Autodesk Inventor part; units mm, degrees
ref_plane "Work Plane1" through (0, 20, 0) normal (0, 1, 0) x (-1, 0, 0)
ref_plane "Work Plane3" through (0, 0, 0) normal (-1, 0, 0) x (0, 0, 1)
ref_plane "YZ Plane" through (0, 0, 0) normal (1, 0, 0) x (0, 1, 0)
sketch "Sketch1" plane through (0, 0, 0) normal (0, 0, 1) x (1, 0, 0)
  line L0 (0, 0) -> (0, 6.5)
  line L1 (0, 6.5) -> (55, 6.5)
  line L2 (68, 1.75) -> (55, 6.5)
  line L3 (72, 0) -> (72, 2.5)
  line L4 (72, 2.5) -> (68, 1.75)
  line L5 (0, 6.5) -> (0, 9.5)
  line L6 (0, 9.5) -> (60.7761, 9.5)
  line L7 (72, 0) -> (0, 0)
  line L8 (72, 2.5) -> (72, 4.5)
  line L9 (72, 4.5) -> (66.9088, 4.5)
  line L10 (66.9088, 4.5) -> (66.9088, 9.5)
  line L11 (66.9088, 9.5) -> (60.7761, 9.5)
  line L12 (66.9088, 9.5) -> (66.9088, 9.5)
  line L13 (66.9088, 9.5) -> (16.9088, 9.5)
  line L14 (16.9088, 9.5) -> (16.9088, 9.5)
  point P0 (72, 1.25)
  dimension "d0" = 6.5
  dimension "d1" = 55
  dimension "d5" = 2.5
  dimension "d6" = 3
  dimension "d7" = 0
  dimension "d8" = 50
  dimension "d44" = 1.75
  dimension "d45" = 4
  dimension "d46" = 13
revolve "Revolution1" add sketch "Sketch1" angle 360 about axis through (72, 0, 0) along (-1, 0, 0) contours L5 L6 L11 L10 L9 L8 L4 L2 L1
sketch "Sketch2" plane through (0, 0, 0) normal (-1, 0, 0) x (0, 0, 1)
  circle A0 centre (0, 0) radius 2.5
  circle A1 centre (0, 0) radius 20
  circle A2 centre (0, 0) radius 6.5
  dimension "d10" = 40
  dimension "d11" = 13
extrude "Extrusion1" add sketch "Sketch2" along normal blind 19 contours A1
sketch "Sketch3" plane through (0, 0, 0) normal (1, 0, 0) x (0, 0, -1)
  circle A0 centre (0, 0) radius 1.75
  circle A1 centre (0, 0) radius 20
  circle A2 centre (0, 0) radius 4.5
  circle A3 centre (0, 0) radius 9.5
  dimension "d18" = 40
  dimension "d37" = 19
extrude "Extrusion2" add sketch "Sketch3" along normal blind 15 contours A1
sketch "Sketch4" plane through (0, 0, 0) normal (0, 1, 0) x (-1, 0, 0)
  line L0 (19, -20) -> (19, 20)
  line L1 (19, 0) -> (-5, 0)
  circle A0 centre (-5, 0) radius 1.75
  point P0 (0, 0)
  dimension "d21" = 24
  dimension "d22" = 3.5
extrude "Extrusion3" cut sketch "Sketch4" along normal through all both and the other way through all
ref_plane "Work Plane1" through (0, 20, 0) normal (0, 1, 0) x (-1, 0, 0)
sketch "Sketch5" plane through (0, 20, 0) normal (0, 1, 0) x (-1, 0, 0)
  line L0 (19, -20) -> (19, 20)
  line L1 (19, 0) -> (-5, 0)
  circle A0 centre (-5, 0) radius 3.175
  point P0 (0, 0)
  dimension "d26" = 24
  dimension "d27" = 6.35
hole "Hole1" at (5, 20, 0) direction (0, -1, 0) diameter 2 end through all counterbore diameter 11 counterbore depth 6
thread "Thread3"
mirror "Mirror1" about plane through (0, 0, 0) normal (0, 1, 0) of "Hole1"
thread "Thread4"
ref_plane "Work Plane3" through (0, 0, 0) normal (-1, 0, 0) x (0, 0, 1)
ref_plane "Work Plane2" through (0, 0, 0) normal (0, 1, 0) x (-1, 0, 0)
properties part number "ASI Propane" material "Stainless Steel"
Read the model definition and answer for the solid it produces. Units are mm, in the model's axes. A direction names the side the tool comes from. Coordinates: 2 decimals unless noted, no trailing zeros. Loops run counter-clockwise (first coordinate to the right, second up) from the corner with the lowest first, then second, coordinate; pieces in that order, holes last.
(1) The part is cut by section A-A (x = 5). Determine the outline of the cut face in (y, z).
Solution:
outline: (-19.23, -5.5) arc R20 ccw to (19.23, -5.5) - (14, -5.5) - (14, -1.75) - (6.26, -1.75) arc R6.5 cw to (-6.26, -1.75) - (-14, -1.75) - (-14, -5.5) - close; (-19.23, 5.5) - (-14, 5.5) - (-14, 1.75) - (-6.26, 1.75) arc R6.5 cw to (6.26, 1.75) - (14, 1.75) - (14, 5.5) - (19.23, 5.5) arc R20 ccw to start
(2) The mould has two halves that part along Y. Classify faces 1 (the face through (-2.238, 19.956, 1.319)), 2 (the face through (18.518, 6.033, 2.419)), 3 (the face through (72, 2, 2)): released by +Y, released by -Y, zero draft, split by the parting line, or undercut.
Solution:
face 1: split by the parting line
face 2: undercut
face 3: zero draft
(3) Flat-ended cylindrical pins translate along their axes: pin 1 Ø5.5 at (x, z) = (5, 0) entering from -Y; pin 2 Ø6.5 at (x, z) = (5, 0) entering from +Y; pin 3 Ø4 at (y, z) = (-6, -6.5) entering from +X; pin 4 Ø17 at (y, z) = (0, 0) entering from -X. Find the tip coordinate at first contact, or state that the pin passes through.
Solution:
pin 1: stops at y = -14
pin 2: stops at y = 14
pin 3: stops at x = 66.91
pin 4: stops at x = -19
(4) Consider line 1 along X through (y, z) = (-11.5, 0); line 2 along Z through (x, y) = (24, 0); line 3 along X through (y, z) = (-7.5, 11.5). Determine where each line is inside the solid, lowest interval first.
Solution:
line 1: x = -19 to 3.25, 6.75 to 15
line 2: z = -9.5 to -6.5, 6.5 to 9.5
line 3: x = -19 to 15
(5) The part is cut by section B-B (x = 26.5). Determine the outline of the cut face in (y, z), and give its area (3 significant figures).
Solution:
outline: circle Ø19 at (0, 0); hole circle Ø13 at (0, 0)
area: 151 mm2
(6) A tool of negligible diameter and unlimited length cuts with its end or side. For faces 4 (the face through (7, -14, 0)), 5 (the face through (7.11, 16.96, 5.08)), 6 (the face through (69.42, -0.59, -4.46)), from which of +Z, -Z, +X, -X, +Y, -Y can it reach the whole face along a straight path? Write none if from no direction.
Solution:
face 4: -Y
face 5: +Y
face 6: +X
